The model under review builds one solid part; all positions refer to its coordinate system, in mm. Face numbers are marked on the shaded views. A direction names the side the tool comes from. Coordinates: 2 decimals unless noted, no trailing zeros. Loops run counter-clockwise (first coordinate to the right, second up) from the corner with the lowest first, then second, coordinate; pieces in that order, holes last. Notation, with made-up numbers: M -24,13 L 26,13 A23 ccw 26,29 Z; hole C 1,-3 d7. An arc over 180 degrees is marked long. Write item = value, one per line. Start each with the question number.
Q1. Mouldability with a two-part tool opening along Z and no side actions: class the marked faces 3, 4 and 5 as released by +Z, released by -Z, zero draft, split by the parting line, or undercut.
Q2. Clearance check with flat-ended pins moving along their axes: pin 1 Ø1.5 at (x, z) = (-5.5, -3.5) entering from -Y; pin 2 Ø1.5 at (x, z) = (2.5, 0) entering from +Y (1 decimal); pin 3 Ø12 at (x, y) = (2, 21.5) entering from +Z; pin 4 Ø6 at (x, y) = (-3.5, 33.5) entering from +Z. State where each tip first meets the part, or that it passes through.
Q3. We need section B-B on z = 0. Count the separate pieces of the cut face and the enclosed holes in it, and give its area (3 significant figures).
Q4. We need section A-A on x = 10. Give the boundary of the cut face in (y, z), and give its area (3 significant figures).
Q5. Wall thickness on probe 1 along Z at (x, y) = (0, 53); probe 2 along Z at (x, y) = (-10, 72.2); probe 3 along Y at (x, z) = (10, -2.5): over which ranges is each line inside the solid? List them lowest first.
Q6. We need section C-C on y = 8. Give the boundary of the cut face in (x, z), and give its area (3 significant figures).
Q7. For the marked faces 1 and 2, list the 3-axis set-ups (+Z, -Z, +X, -X, +Y, -Y) from which the entire face can be reached by the end or side of a thin tool; tool diameter is ignored.
Autodesk Inventor part; units mm, degrees
ref_plane "YZ Plane" through (0, 0, 0) normal (1, 0, 0) x (0, 1, 0)
ref_plane "XZ Plane" through (0, 0, 0) normal (0, 1, 0) x (-1, 0, 0)
ref_plane "XY Plane" through (0, 0, 0) normal (0, 0, 1) x (1, 0, 0)
sketch "Sketch1" plane through (0, 0, 0) normal (0, 1, 0) x (-1, 0, 0)
  circle A0 centre (0, 0) radius 4.35
  circle A1 centre (0, 0) radius 7.5
  dimension "d0" = 8.7
  dimension "d4" = 15
extrude "Extrusion1" add sketch "Sketch1" along normal blind 75
sketch "Sketch2" plane through (0, 75, 0) normal (0, 1, 0) x (1, 0, 0)
  circle A0 centre (-10, 0) radius 1.5
  circle A1 centre (10, 0) radius 1.5
  circle A2 centre (-10, 0) radius 3
  circle A3 centre (10, 0) radius 3
  point P0 (0, 0)
  dimension "d8" = 3
  dimension "d9" = 20
  dimension "d10" = 10
  dimension "d11" = 6
extrude "Extrusion2" add sketch "Sketch2" against normal blind 6
fillet "Fillet1" radius 2 4 edges at (-7.3625, 72, -1.4295) (-7.3625, 72, 1.4295) (7.3625, 72, -1.4295) (7.3625, 72, 1.4295)
sketch "Sketch3" plane through (0, 0, 0) normal (0, -1, 0) x (1, 0, 0)
  circle A0 centre (0, 0) radius 6.5
  circle A1 centre (0, 0) radius 6.5
  circle A2 centre (0, 0) radius 7.5
  circle A3 centre (0, 0) radius 7.5
  dimension "d15" = 13
extrude "Extrusion3" cut sketch "Sketch3" against normal blind 55
sketch "Sketch4" plane through (0, 0, 0) normal (0, -1, 0) x (1, 0, 0)
  circle A0 centre (0, 0) radius 5.5
  circle A1 centre (0, 0) radius 6.5
  circle A2 centre (0, 0) radius 6.5
  dimension "d18" = 11
extrude "Extrusion4" cut sketch "Sketch4" against normal blind 28
chamfer "Chamfer2" distance 1 angle 45 3 edges at (7.5, 55, 0) (-6.5, 28, 0) (-5.5, 0, 0)
properties part number "Spacer"
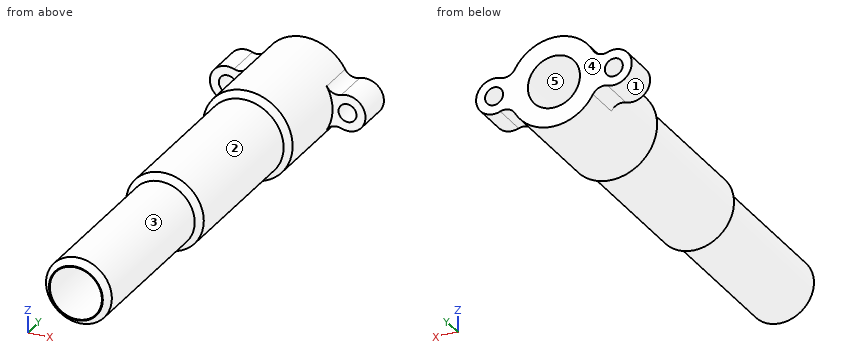
Returned:
q1.face_3 = split by the parting line
q1.face_4 = zero draft
q1.face_5 = undercut
q2.pin_1 = 28.27
q2.pin_2 = through
q2.pin_3 = 5.5
q2.pin_4 = 6.48
q3.separate_pieces = 4
q3.enclosed_holes = 0
q3.area = 334 mm^2
q4.outline = M 69,-3 L 75,-3 L 75,-1.5 L 69,-1.5 Z; M 69,1.5 L 75,1.5 L 75,3 L 69,3 Z
q4.area = 18.0 mm^2
q5.probe_1 = -6.5 to -4.35, 4.35 to 6.5
q5.probe_2 = -3 to -1.5, 1.5 to 3
q5.probe_3 = 69 to 75
q6.outline = C 0,0 d11; hole C 0,0 d8.7
q6.area = 35.6 mm^2
q7.face_1 = +Y, -Y
q7.face_2 = -Y
